Design review of the part built by this model. Coordinates are the model's own, in mm. Give positions to 0.01 mm unless a question says otherwise; leave off trailing zeros. Write each loop counter-clockwise with the first axis right and the second up, starting at its lowest first coordinate (ties: lowest second). Pieces come first, ordered by that corner, then holes.
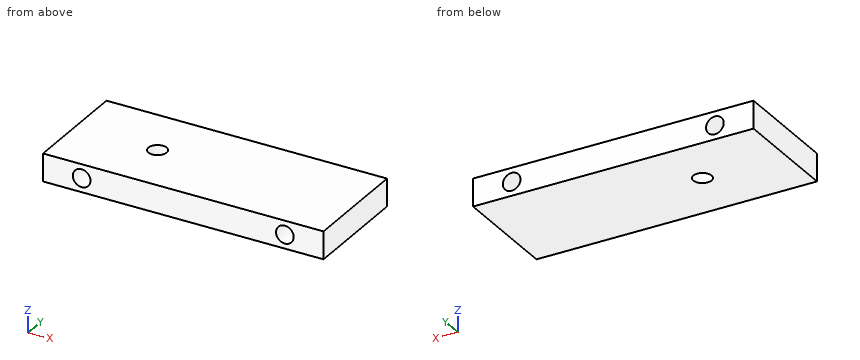
```python
from build123d import *

# Parameters (mm, degrees)
ESQUISSE1_W             = 50.8
ESQUISSE1_H             = 19.9
EXTRUSION1_DEPTH        = 5
TROU_TARAUD_M4X0_71_D   = 3.3
ESQUISSE4_R             = 1.6
ENL_V_MAT_EXTRU_1_DEPTH = 42.263179713


with BuildPart() as part:
    # Esquisse1 → Extrusion1 (new body)
    with BuildSketch(Plane.XY):
        with Locations((10.4, 9.95)):
            Rectangle(ESQUISSE1_W, ESQUISSE1_H)
    extrude(amount=EXTRUSION1_DEPTH)

    # Trou taraudé M4x0.71 (through all)
    with Locations(Plane.XY.offset(5)):
        with Locations((0, 9.95)):
            Hole(TROU_TARAUD_M4X0_71_D / 2)

    # Esquisse4 → Enlèv. mat.-Extru.1 (cut, through all)
    with BuildSketch(Plane(origin=(0, 19.9, 0), x_dir=(1, 0, 0), z_dir=(0, 1, 0))):
        with Locations(Location((-8, -2.5, 0), (0, 0, 270))):
            Circle(ESQUISSE4_R)
        with Locations(Location((28.8, -2.5, 0), (0, 0, 270))):
            Circle(ESQUISSE4_R)
    extrude(amount=-ENL_V_MAT_EXTRU_1_DEPTH, mode=Mode.SUBTRACT)


solid = part.part
```
(1) Consider section D-D, the plane y = 6. Give the boundary of the cut face in (x, z).
Resolved:
outline: (-15, 0) - (35.8, 0) - (35.8, 5) - (-15, 5) - close; hole circle Ø3.2 at (-8, 2.5); hole circle Ø3.2 at (28.8, 2.5)
(2) Consider section A-A, the plane z = 2.5. Give the boundary of the cut face in (x, y).
Resolved:
outline: (-15, 0) - (-9.6, 0) - (-9.6, 19.9) - (-15, 19.9) - close; (-6.4, 0) - (27.2, 0) - (27.2, 19.9) - (-6.4, 19.9) - close; (30.4, 0) - (35.8, 0) - (35.8, 19.9) - (30.4, 19.9) - close; hole circle Ø3.3 at (0, 9.95)
(3) Consider section C-C, the plane y = 9.95. Give the boundary of the cut face in (x, z).
Resolved:
outline: (-15, 0) - (-1.65, 0) - (-1.65, 5) - (-15, 5) - close; (1.65, 0) - (35.8, 0) - (35.8, 5) - (1.65, 5) - close; hole circle Ø3.2 at (-8, 2.5); hole circle Ø3.2 at (28.8, 2.5)
(4) Consider section B-B, the plane x = 0. Give the boundary of the cut face in (y, z), then the cut area to 3 significant figures.
Resolved:
outline: (0, 0) - (8.3, 0) - (8.3, 5) - (0, 5) - close; (11.6, 0) - (19.9, 0) - (19.9, 5) - (11.6, 5) - close
area: 83.0 mm2
(5) To check wall thickness, follow L1, parallel to X at y = 7, z = 2.5; L2, parallel to X at y = 10, z = 2.5; L3, parallel to Y at x = 0, z = 1.6. State the ranges of each line that lie inside material, in increasing order.
Resolved:
L1: x = -15 to -9.6, -6.4 to 27.2, 30.4 to 35.8
L2: x = -15 to -9.6, -6.4 to -1.65, 1.65 to 27.2, 30.4 to 35.8
L3: y = 0 to 8.3, 11.6 to 19.9
(6) Clearance check with flat-ended pins moving along their axes: P1, Ø3, axis at x = 28.8, z = 2.5, coming from the +Y side; P2, Ø1.5, axis at x = 13.5, y = 16.5, coming from the -Z side. State where each tip first meets the part, or that it passes through.
Resolved:
P1: passes through
P2: stops at z = 0
